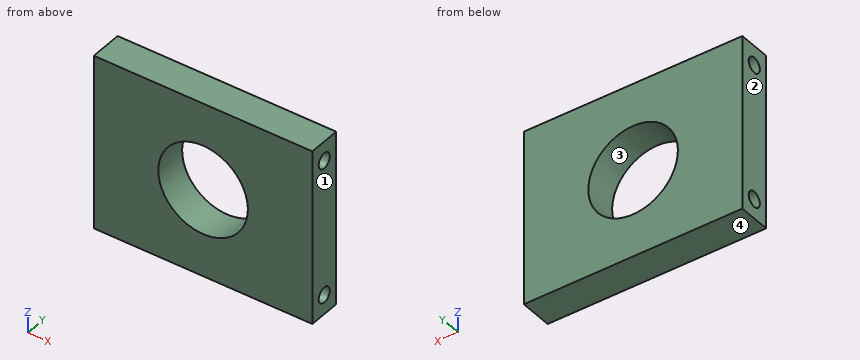
```python
from build123d import *

# Parameters (mm, degrees)
SKETCH1_W           = 100
SKETCH1_H           = 80
SKETCH1_R           = 20.5
BOSS_EXTRUDE1_DEPTH = 15
SKETCH2_R           = 3.5
CUT_EXTRUDE1_DEPTH  = 100


with BuildPart() as part:
    # Sketch1 → Boss-Extrude1 (new body)
    with BuildSketch(Plane(origin=(0, 0, 0), x_dir=(1, 0, 0), z_dir=(0, 1, 0))):
        Rectangle(SKETCH1_W, SKETCH1_H)
        with Locations(Location((0, 0, 0), (0, 0, 270))):
            Circle(SKETCH1_R, mode=Mode.SUBTRACT)
    extrude(amount=BOSS_EXTRUDE1_DEPTH)

    # Sketch2 → Cut-Extrude1 (cut)
    with BuildSketch(Plane(origin=(50, 0, 0), x_dir=(0, 0, -1), z_dir=(1, 0, 0))):
        with Locations((-31.091464528, 7.5)):
            Circle(SKETCH2_R)
        with Locations(Location((31.091464528, 7.5, 0), (0, 0, 180))):
            Circle(SKETCH2_R)
    extrude(amount=-CUT_EXTRUDE1_DEPTH, mode=Mode.SUBTRACT)


solid = part.part
```
Could you check a few things on this model? Use its own coordinates, in mm. Face numbers are marked on the shaded views. Round coordinates to 2 decimals unless told otherwise and drop trailing zeros. Loops run counter-clockwise (first coordinate to the right, second up) from the corner with the lowest first, then second, coordinate; pieces in that order, holes last. Notation, with made-up numbers: M 27,47 L 80,47 A9 cw 80,51 Z; hole C 80,69 d10. An arc over 180 degrees is marked long. Write item = value, one per line.
1. Will this pin go through, and if not, where does the flat tip stop? P1, Ø5.5, axis at y = 7.5, z = 31.09, coming from the +X side.
Results below:
P1 = through
2. I want a section at C-C, the plane z = 0. Write out the boundary of the cut face in (x, y).
Results below:
outline = M -50,0 L -20.5,0 L -20.5,15 L -50,15 Z; M 20.5,0 L 50,0 L 50,15 L 20.5,15 Z
3. Thinking about a two-plate mould opening in X: for the marked faces 1, 2, 3 and 4, which applies, +X half, -X half, draft (parallel to the pull), parting line (faces both ways), or undercut?
Results below:
face_1 = +X half
face_2 = -X half
face_3 = undercut
face_4 = draft
4. I need wall thicknesses on probe 1 along Z at (x, y) = (44.5, 5); probe 2 along X at (y, z) = (12.5, 9); probe 3 along Y at (x, z) = (33.5, -30.5). Which ranges of each line are inside material? Lowest first, please.
Results below:
probe_1 = -40 to -33.54, -28.64 to 28.64, 33.54 to 40
probe_2 = -50 to -18.42, 18.42 to 50
probe_3 = 0 to 4.05, 10.95 to 15
5. I want a section at B-B, the plane x = 0. Write out the boundary of the cut face in (y, z), and give its area (3 significant figures).
Results below:
outline = M 0,-40 L 15,-40 L 15,-20.5 L 0,-20.5 Z; M 0,20.5 L 15,20.5 L 15,40 L 0,40 Z; hole C 7.5,-31.09 d7; hole C 7.5,31.09 d7
area = 508 mm²
6. I want a section at D-D, the plane y = 13. Write out the boundary of the cut face in (x, z).
Results below:
outline = M -50,-40 L 50,-40 L 50,40 L -50,40 Z; hole C 0,0 d41
7. I want a section at A-A, the plane y = 7.5. Write out the boundary of the cut face in (x, z), and give its area (3 significant figures).
Results below:
outline = M -50,-40 L 50,-40 L 50,-34.59 L -50,-34.59 Z; M -50,-27.59 L 50,-27.59 L 50,27.59 L -50,27.59 Z; M -50,34.59 L 50,34.59 L 50,40 L -50,40 Z; hole C 0,0 d41
area = 5,280 mm²
